Design review of the part built by this model. Coordinates are the model's own, in mm. Face numbers are marked on the shaded views. Round coordinates to 2 decimals unless told otherwise and drop trailing zeros. Write each loop counter-clockwise with the first axis right and the second up, starting at its lowest first coordinate (ties: lowest second). Pieces come first, ordered by that corner, then holes. Notation, with made-up numbers: (73.5, 61.5) -> (108.5, 61.5) arc R23 ccw to (108.5, 88.5) -> close; hole circle Ø2 at (12, -30.5). An arc over 180 degrees is marked (long way). Write item = value, one per line. Start each with the question number.
Item 1: Add section A-A, the plane x = 0. State the section outline as (y, z) points.
Item 2: Mouldability with a two-part tool opening along Z and no side actions: class the marked faces 1, 2, 3 and 4 as released by +Z, released by -Z, zero draft, split by the parting line, or undercut.
Item 3: To check wall thickness, follow L1, parallel to X at y = 8.8, z = 0; L2, parallel to Z at x = 18.25, y = 8; L3, parallel to X at y = -2.5, z = 0. State the ranges of each line that lie inside material, in increasing order.
Item 4: Add section B-B, the plane z = 0. State the section outline as (x, y) points, then the cut area to 3 significant figures.
Item 5: Add section C-C, the plane y = -5.5. State the section outline as (x, z) points.
Item 6: For pin 1 Ø7 at (x, z) = (0, 0) entering from -Y; pin 2 Ø2.5 at (x, z) = (17.5, 0) entering from +Y, all flat-tipped, find the tip position at first contact; note any pin that passes through.
Item 7: Add section D-D, the plane x = -18.25. State the section outline as (y, z) points.
from build123d import *

# Parameters (mm, degrees)
SKETCH2_W           = 60
SKETCH2_H           = 20
BOSS_EXTRUDE1_DEPTH = 13.5
SKETCH3_R           = 2.5
CUT_EXTRUDE1_DEPTH  = 3
SKETCH4_R           = 4
CUT_EXTRUDE2_DEPTH  = 39.5


with BuildPart() as part:
    # Sketch2 → Boss-Extrude1 (new, symmetric)
    with BuildSketch(Plane.XY):
        Rectangle(SKETCH2_W, SKETCH2_H)
    extrude(amount=BOSS_EXTRUDE1_DEPTH, both=True)

    # Sketch3 → Cut-Extrude1 (cut)
    with BuildSketch(Plane(origin=(0, 10, 0), x_dir=(1, 0, 0), z_dir=(0, 1, 0))):
        with Locations(Location((-18.25, 0, 0), (0, 0, 270))):
            Circle(SKETCH3_R)
        with Locations(Location((18.25, 0, 0), (0, 0, 90))):
            Circle(SKETCH3_R)
    extrude(amount=-CUT_EXTRUDE1_DEPTH, mode=Mode.SUBTRACT)

    # Sketch4 → Cut-Extrude2 (cut, through all)
    with BuildSketch(Plane(origin=(0, 10, 0), x_dir=(1, 0, 0), z_dir=(0, 1, 0))):
        with Locations(Location((0, 0, 0), (0, 0, 270))):
            Circle(SKETCH4_R)
    extrude(amount=-CUT_EXTRUDE2_DEPTH, mode=Mode.SUBTRACT)


solid = part.part
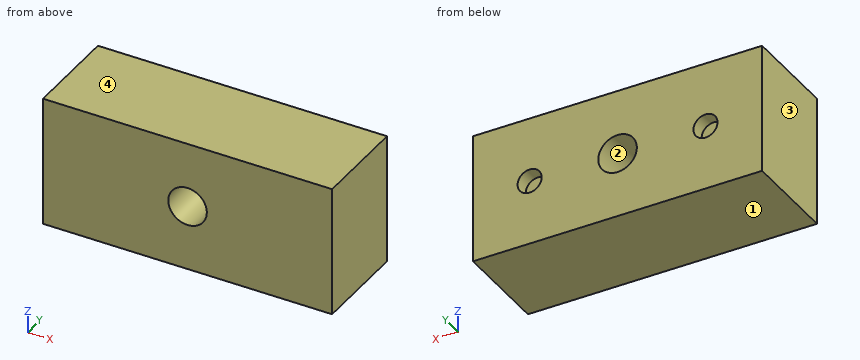
Result set:
q1.outline = (-10, -13.5) -> (10, -13.5) -> (10, -4) -> (-10, -4) -> close; (-10, 4) -> (10, 4) -> (10, 13.5) -> (-10, 13.5) -> close
q2.face_1 = released by -Z
q2.face_2 = undercut
q2.face_3 = zero draft
q2.face_4 = released by +Z
q3.L1 = -30 to -20.75, -15.75 to -4, 4 to 15.75, 20.75 to 30
q3.L2 = -13.5 to -2.5, 2.5 to 13.5
q3.L3 = -30 to -4, 4 to 30
q4.outline = (-30, -10) -> (-4, -10) -> (-4, 10) -> (-15.75, 10) -> (-15.75, 7) -> (-20.75, 7) -> (-20.75, 10) -> (-30, 10) -> close; (4, -10) -> (30, -10) -> (30, 10) -> (20.75, 10) -> (20.75, 7) -> (15.75, 7) -> (15.75, 10) -> (4, 10) -> close
q4.area = 1,010 mm²
q5.outline = (-30, -13.5) -> (30, -13.5) -> (30, 13.5) -> (-30, 13.5) -> close; hole circle Ø8 at (0, 0)
q6.pin_1 = through
q6.pin_2 = 7
q7.outline = (-10, -13.5) -> (10, -13.5) -> (10, -2.5) -> (7, -2.5) -> (7, 2.5) -> (10, 2.5) -> (10, 13.5) -> (-10, 13.5) -> close
